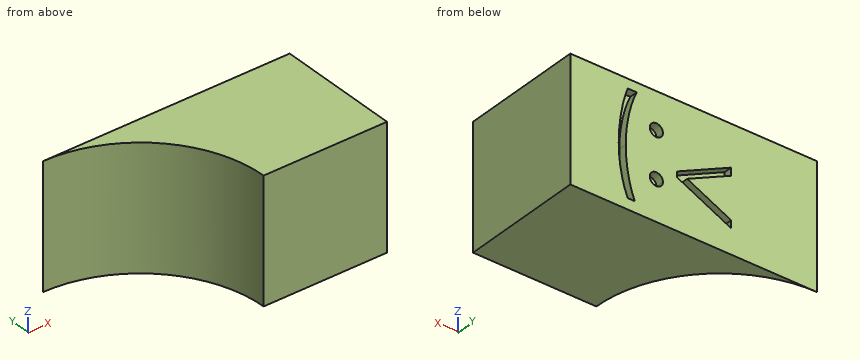
```python
from build123d import *

# Parameters (mm, degrees)
SKETCH1_W           = 30
SKETCH1_H           = 15
BOSS_EXTRUDE1_DEPTH = 15
SKETCH2_R           = 15
CUT_EXTRUDE1_DEPTH  = 15
CUT_EXTRUDE2_DEPTH  = 1


with BuildPart() as part:
    # Sketch1 → Boss-Extrude1 (new body)
    with BuildSketch(Plane(origin=(0, 0, 0), x_dir=(1, 0, 0), z_dir=(0, 1, 0))):
        Rectangle(SKETCH1_W, SKETCH1_H)
    extrude(amount=BOSS_EXTRUDE1_DEPTH)

    # Sketch2 → Cut-Extrude1 (cut)
    with BuildSketch(Plane.XY.offset(7.5)):
        with Locations((-15, 0)):
            Circle(SKETCH2_R)
    extrude(amount=-CUT_EXTRUDE1_DEPTH, mode=Mode.SUBTRACT)

    # Sketch3 → Cut-Extrude2 (cut)
    with BuildSketch(Plane(origin=(0, 15, 0), x_dir=(1, 0, 0), z_dir=(0, 1, 0))):
        Polygon((-4.565210898, -1.540580661), (0.781153285, 1.010486046), (-4.565210898, 3.561552753), (-4.565210898, 4.490774507), (2.029019871, 1.344395301), (2.029019871, 0.676576791), (-4.565210898, -2.469802416), align=None)
        with BuildLine():
            add(Edge.make_bspline(
                [(4.532385256, 3.391736046), (4.585426476, 3.388584178), (4.689407588, 3.382405309), (4.83973693, 3.340014504), (4.975793825, 3.264743436), (5.096985148, 3.164424017), (5.196879202, 3.042787963), (5.274832761, 2.90781624), (5.316854299, 2.756228334), (5.322988159, 2.651644719), (5.326135256, 2.597986046)],
                knots=[0, 0, 0, 0, 0.000159102, 0.000311902, 0.000463876, 0.000622429, 0.000780981, 0.000933875, 0.001086674, 0.001247676, 0.001247676, 0.001247676, 0.001247676], degree=3))
            add(Edge.make_bspline(
                [(5.326135256, 2.597986046), (5.322988159, 2.544327373), (5.316854299, 2.439743758), (5.274832761, 2.288155852), (5.196879202, 2.153184129), (5.096985148, 2.031548075), (4.975793825, 1.931228656), (4.83973693, 1.855957587), (4.689407588, 1.813566782), (4.585426476, 1.807387914), (4.532385256, 1.804236046)],
                knots=[0, 0, 0, 0, 0.000161002, 0.000313801, 0.000466695, 0.000625248, 0.0007838, 0.000935775, 0.001088574, 0.001247676, 0.001247676, 0.001247676, 0.001247676], degree=3))
            add(Edge.make_bspline(
                [(4.532385256, 1.804236046), (4.479307324, 1.807283761), (4.375865992, 1.813223325), (4.226079814, 1.856876161), (4.089202284, 1.930531062), (3.968032593, 2.03173365), (3.867325054, 2.152555772), (3.792822649, 2.289085596), (3.747168888, 2.439306024), (3.741525683, 2.54423952), (3.738635256, 2.597986046)],
                knots=[0, 0, 0, 0, 0.000159102, 0.000310068, 0.000463722, 0.000622275, 0.000780827, 0.000932802, 0.001086136, 0.001247138, 0.001247138, 0.001247138, 0.001247138], degree=3))
            add(Edge.make_bspline(
                [(3.738635256, 2.597986046), (3.741631063, 2.650449237), (3.747548948, 2.754084477), (3.792844046, 2.903037506), (3.867230597, 3.039722332), (3.96867028, 3.160258542), (4.088470126, 3.2638968), (4.226513734, 3.336529736), (4.375479803, 3.383381479), (4.479237718, 3.388906159), (4.532385256, 3.391736046)],
                knots=[0, 0, 0, 0, 0.000157203, 0.000310538, 0.000462512, 0.000621065, 0.000780841, 0.000934495, 0.001086002, 0.001245105, 0.001245105, 0.001245105, 0.001245105], degree=3))
        make_face()
        with BuildLine():
            add(Edge.make_bspline(
                [(4.532385256, -2.225571646), (4.585426476, -2.228723514), (4.689407588, -2.234902383), (4.83973693, -2.277293188), (4.975793825, -2.352564257), (5.096985148, -2.452883675), (5.196879202, -2.57451973), (5.274832761, -2.709491453), (5.316854299, -2.861079358), (5.322988159, -2.965662974), (5.326135256, -3.019321646)],
                knots=[0, 0, 0, 0, 0.000159102, 0.000311902, 0.000463876, 0.000622429, 0.000780981, 0.000933875, 0.001086674, 0.001247676, 0.001247676, 0.001247676, 0.001247676], degree=3))
            add(Edge.make_bspline(
                [(5.326135256, -3.019321646), (5.322881514, -3.071690994), (5.316465182, -3.174962578), (5.274929085, -3.32540713), (5.196285105, -3.460463205), (5.09767416, -3.583749738), (4.975763866, -3.684281679), (4.839415269, -3.758912353), (4.689760488, -3.804338384), (4.585485351, -3.81012495), (4.532385256, -3.813071646)],
                knots=[0, 0, 0, 0, 0.000157203, 0.000310002, 0.000462897, 0.000622923, 0.000781475, 0.00093345, 0.001086785, 0.001245887, 0.001245887, 0.001245887, 0.001245887], degree=3))
            add(Edge.make_bspline(
                [(4.532385256, -3.813071646), (4.479246898, -3.810231571), (4.375506905, -3.804687001), (4.226410735, -3.757979649), (4.08923177, -3.684981518), (3.967345212, -3.583562286), (3.867908372, -3.46109761), (3.792727865, -3.324477007), (3.74757896, -3.175393238), (3.741641149, -3.071775817), (3.738635256, -3.019321646)],
                knots=[0, 0, 0, 0, 0.000159102, 0.000310609, 0.000464264, 0.000622816, 0.000782843, 0.000934817, 0.001088152, 0.001245355, 0.001245355, 0.001245355, 0.001245355], degree=3))
            add(Edge.make_bspline(
                [(3.738635256, -3.019321646), (3.741525683, -2.96557512), (3.747168888, -2.860641624), (3.792822649, -2.710421196), (3.867325054, -2.573891372), (3.968032593, -2.453069251), (4.089202284, -2.351866663), (4.226079814, -2.278211761), (4.375865992, -2.234558925), (4.479307324, -2.228619362), (4.532385256, -2.225571646)],
                knots=[0, 0, 0, 0, 0.000161002, 0.000314336, 0.000466311, 0.000624863, 0.000783415, 0.00093707, 0.001088035, 0.001247138, 0.001247138, 0.001247138, 0.001247138], degree=3))
        make_face()
        with BuildLine():
            Line((8.012673717, -6.377494723), (6.913635256, -6.377494723))
            add(Edge.make_bspline(
                [(6.913635256, -6.377494723), (6.964923037, -6.268556916), (7.068946293, -6.047606327), (7.207381282, -5.703499581), (7.344635711, -5.34898027), (7.470061478, -4.979429934), (7.587529774, -4.596798161), (7.699577806, -4.200923285), (7.798655827, -3.790991301), (7.927768443, -3.226973351), (8.061537871, -2.505405036), (8.172348909, -1.623616401), (8.244020266, -0.728938898), (8.252595321, -0.127485519), (8.256904487, 0.174758882)],
                knots=[0, 0, 0, 0, 0.000361147, 0.000732487, 0.001112362, 0.001501554, 0.001902903, 0.002313081, 0.002735593, 0.00316793, 0.004048889, 0.004935676, 0.005833185, 0.006739799, 0.006739799, 0.006739799, 0.006739799], degree=3))
            add(Edge.make_bspline(
                [(8.256904487, 0.174758882), (8.252902226, 0.454678656), (8.244972319, 1.009299641), (8.191798742, 1.834123368), (8.097085547, 2.6424037), (7.970871979, 3.430798715), (7.811358038, 4.187699516), (7.62592252, 4.903463701), (7.412126188, 5.57256258), (7.24119411, 5.994633525), (7.157866025, 6.200389892)],
                knots=[0, 0, 0, 0, 0.00083976, 0.001663864, 0.002478263, 0.003280358, 0.00405836, 0.004797909, 0.005497855, 0.006163637, 0.006163637, 0.006163637, 0.006163637], degree=3))
            Line((7.157866025, 6.200389892), (8.012673717, 6.200389892))
            add(Edge.make_bspline(
                [(8.012673717, 6.200389892), (8.054744003, 6.10338045), (8.139913324, 5.90698938), (8.256148684, 5.601782231), (8.365580554, 5.284503822), (8.472030365, 4.95493584), (8.568429545, 4.612298427), (8.65782742, 4.256424857), (8.742333903, 3.88830928), (8.843284081, 3.378212649), (8.953267541, 2.726122679), (9.043476277, 1.92739898), (9.100527601, 1.113721058), (9.107966351, 0.565368415), (9.111712179, 0.289242056)],
                knots=[0, 0, 0, 0, 0.000317185, 0.000642126, 0.000979441, 0.001323997, 0.001680966, 0.002047019, 0.002424721, 0.002813889, 0.003606878, 0.00440779, 0.005224405, 0.00605272, 0.00605272, 0.00605272, 0.00605272], degree=3))
            add(Edge.make_bspline(
                [(9.111712179, 0.289242056), (9.108657505, -0.008500857), (9.10258886, -0.600019428), (9.046302547, -1.482164848), (8.960344753, -2.353183983), (8.835781357, -3.209818768), (8.680204435, -4.045048948), (8.494446198, -4.852986274), (8.274075254, -5.629424741), (8.099072178, -6.130242561), (8.012673717, -6.377494723)],
                knots=[0, 0, 0, 0, 0.000893134, 0.001774367, 0.002650754, 0.003518288, 0.004370411, 0.005198895, 0.006004563, 0.006790171, 0.006790171, 0.006790171, 0.006790171], degree=3))
        make_face()
    extrude(amount=-CUT_EXTRUDE2_DEPTH, mode=Mode.SUBTRACT)


solid = part.part
```
Could you check a few things on this model? Use its own coordinates, in mm. Coordinates: 2 decimals unless noted, no trailing zeros. Order: outer loops, then holes, each group sorted by start corner. A loop starts at its lowest first (then second) coordinate and runs counter-clockwise, first axis right, second up. Notation, with made-up numbers: M 22,0 L 37,0 A9 cw 37,10 Z; hole C 30,75 d10. An arc over 180 degrees is marked long. Use one line per item in the form item = value. Start each with the question number.
1. Suppose I cut it at A-A on x = -4. Write out the boundary of the cut face in (y, z), then the cut area to 3 significant figures.
2. Please list where these lines run through material, in increasing order: line 1 (X direction, y = 8, z = -5); line 2 (Y direction, x = -5.5, z = -1.5); line 3 (X direction, y = 6.25, z = 3).
3. For pin 1 (5 mm diameter, centred on x = 12, z = 0, fed in from -Y); pin 2 (4 mm diameter, centred on x = -9, z = -2, fed in from -Y); pin 3 (4 mm diameter, centred on y = 10.5, z = -2.5, fed in from -X), each with a flat end and sliding along its axis, tell me the tip position at first contact or that it passes through.
4. Suppose I cut it at B-B on y = 9. Write out the boundary of the cut face in (x, z), then the cut area to 3 significant figures.
5. Suppose I cut it at D-D on y = 5.5. Write out the boundary of the cut face in (x, z), then the cut area to 3 significant figures.
6. Suppose I cut it at C-C on x = -0.5. Write out the boundary of the cut face in (y, z), then the cut area to 3 significant figures.
Geometry says:
q1.outline = M 10.2,-7.5 L 15,-7.5 L 15,-4.22 L 14,-4.22 L 14,-3.29 L 15,-3.29 L 15,1.27 L 14,1.27 L 14,2.2 L 15,2.2 L 15,7.5 L 10.2,7.5 Z
q1.area = 70.2 mm^2
q2.line_1 = -2.31 to 15
q2.line_2 = 11.61 to 15
q2.line_3 = -1.36 to 15
q3.pin_1 = 0
q3.pin_2 = 12.69
q3.pin_3 = -6.71
q4.outline = M -3,-7.5 L 15,-7.5 L 15,7.5 L -3,7.5 Z
q4.area = 270 mm^2
q5.outline = M -1.04,-7.5 L 15,-7.5 L 15,7.5 L -1.04,7.5 Z
q5.area = 241 mm^2
q6.outline = M 3.84,-7.5 L 15,-7.5 L 15,-2.55 L 14,-2.55 L 14,-1.62 L 15,-1.62 L 15,-0.4 L 14,-0.4 L 14,0.53 L 15,0.53 L 15,7.5 L 3.84,7.5 Z
q6.area = 166 mm^2
